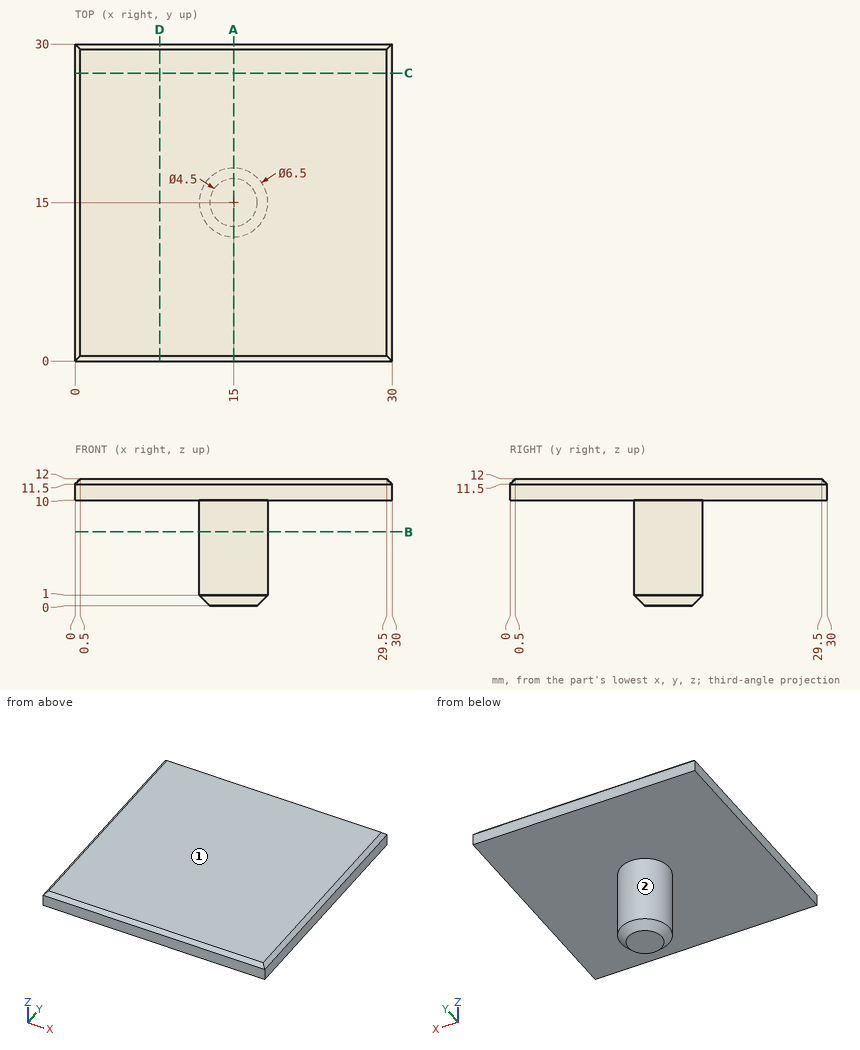
Answer from the drawing. Dimensions are ordinates in mm from the lowest x, y and z of the part. A direction names the side the tool comes from. Round coordinates to 2 decimals unless told otherwise and drop trailing zeros. Loops run counter-clockwise (first coordinate to the right, second up) from the corner with the lowest first, then second, coordinate; pieces in that order, holes last.
Q1. Which of the six approach directions +Z, -Z, +X, -X, +Y, -Y give full straight-line access (tool end or side, diameter ignored) to the marked faces 1 and 2?
Q2. Section C-C on y = 27.25 is taken. Write down the section's boundary in (x, z).
Q3. This flat-tipped pin is pushed along its axis until it touches: pin 1 (1.5 mm diameter, centred on x = 17.5, y = 7.5, fed in from -Z). Where does it stop, or does it pass through?
Q4. Section B-B on z = 7 is taken. Write down the section's boundary in (x, y).
Q5. Consider probe 1 along Z at (x, y) = (19.25, 3.75); probe 2 along Y at (x, z) = (12.5, 3.75); probe 3 along Y at (x, z) = (17, 8). Determine where each line is inside the solid, lowest interval first.
Q6. Section A-A on x = 15 is taken. Write down the section's boundary in (y, z), and give its area (3 significant figures).
Output:
1. face 1: +Z, +X, -X, +Y, -Y
1. face 2: -Z
2. outline: (0, 10) - (30, 10) - (30, 11.5) - (29.5, 12) - (0.5, 12) - (0, 11.5) - close
3. pin 1: stops at z = 10
4. outline: circle Ø6.5 at (15, 15)
5. probe 1: z = 10 to 12
5. probe 2: y = 12.92 to 17.08
5. probe 3: y = 12.44 to 17.56
6. outline: (0, 10) - (11.75, 10) - (11.75, 1) - (12.75, 0) - (17.25, 0) - (18.25, 1) - (18.25, 10) - (30, 10) - (30, 11.5) - (29.5, 12) - (0.5, 12) - (0, 11.5) - close
6. area: 124 mm2
